Source: CAD feature listing. Evaluate the final solid. Frame: model axes, mm. A direction names the side the tool comes from. Coordinates: 2 decimals unless noted, no trailing zeros. Order: outer loops, then holes, each group sorted by start corner. A loop starts at its lowest first (then second) coordinate and runs counter-clockwise, first axis right, second up.
Item 1: Section B-B on x = 17. Return the cut outline in (y, z), then the cut area to 4 significant figures.
Item 2: Reachability of faces 1 (the flat face through (0, 2, 20)), 2 (the cylindrical face through (-0.74, 10.9, -3.32)), 3 (the flat face through (0, 2, -20)), 4 (the flat face through (0, -3.5, 0)) from +Z, -Z, +X, -X, +Y, -Y: full face, straight path, thin tool, end or side. Return the list, or none.
Item 3: Ray query, line 1 (Y direction, x = -17, z = -22); line 2 (Y direction, x = -10, z = 6.5); line 3 (X direction, y = 10.75, z = -0.5). Return the intervals inside material, ascending.
Item 4: Section A-A on z = 0. Return the cut outline in (x, y), then the cut area to 3 significant figures.
Item 5: Section C-C on y = 1. Return the cut outline in (x, z).
Item 6: Contact query for flat-ended pins moving along their axis: P1, Ø3, axis at x = -9, z = 21, coming from the +Y side; P2, Ø1, axis at x = -2.5, y = 2.5, coming from the -Z side; P3, Ø1, axis at x = -5.5, y = 1.5, coming from the +Z side. Output: stop coordinate, or through.
Item 7: Section D-D on x = 0. Return the cut outline in (y, z).
Autodesk Inventor part; units mm, degrees
ref_plane "YZ Plane" through (0, 0, 0) normal (1, 0, 0) x (0, 1, 0)
ref_plane "XZ Plane" through (0, 0, 0) normal (0, 1, 0) x (-1, 0, 0)
ref_plane "XY Plane" through (0, 0, 0) normal (0, 0, 1) x (1, 0, 0)
sketch "Sketch1" plane through (0, 0, 0) normal (0, 1, 0) x (-1, 0, 0)
  line L0 (20, 20) -> (-20, 20)
  line L1 (-20, 20) -> (-20, -20)
  line L2 (-20, -20) -> (20, -20)
  line L3 (20, -20) -> (20, 20)
  point P0 (0, 0)
  point P1 (20, 0)
  point P2 (0, -20)
  dimension "d0" = 40
  dimension "d1" = 40
extrude "Extrusion1" add sketch "Sketch1" along normal blind 3.5
sketch "Sketch2" plane through (0, 0, 0) normal (0, -1, 0) x (1, 0, 0)
  line L0 (20, 23.5) -> (-20, 23.5)
  line L1 (-20, 23.5) -> (-20, -23.5)
  line L2 (-20, -23.5) -> (20, -23.5)
  line L3 (20, -23.5) -> (20, 23.5)
  line L4 (20, 20) -> (20, -20)
  line L5 (20, -20) -> (-20, -20)
  point P0 (0, 0)
  point P1 (0, -23.5)
  point P2 (20, 0)
  dimension "d5" = 3.5
extrude "Extrusion2" add sketch "Sketch2" along normal blind 3.5
sketch "Sketch3" plane through (0, 3.5, 0) normal (0, 1, 0) x (1, 0, 0)
  line L0 (-12.5, 12.5) -> (12.5, 12.5)
  line L1 (12.5, 12.5) -> (12.5, -12.5)
  line L2 (12.5, -12.5) -> (-12.5, -12.5)
  line L3 (-12.5, -12.5) -> (-12.5, 12.5)
  circle A0 centre (0, 0) radius 3.4
  point P0 (12.5, 0)
  point P1 (0, 12.5)
  dimension "d8" = 25
  dimension "d9" = 25
  dimension "d12" = 6.8
extrude "Extrusion4" add sketch "Sketch3" along normal blind 15 contours A0
properties part number "Einschub"
Answer list:
1. outline: (-3.5, -23.5) - (0, -23.5) - (0, -20) - (3.5, -20) - (3.5, 20) - (0, 20) - (0, 23.5) - (-3.5, 23.5) - close
1. area: 304.5 mm2
2. face 1: +Z, +X, -X, +Y
2. face 2: +Y
2. face 3: -Z, +X, -X, +Y
2. face 4: +Z, -Z, +X, -X, -Y
3. line 1: y = -3.5 to 0
3. line 2: y = -3.5 to 3.5
3. line 3: x = -3.36 to 3.36
4. outline: (-20, -3.5) - (20, -3.5) - (20, 3.5) - (3.4, 3.5) - (3.4, 18.5) - (-3.4, 18.5) - (-3.4, 3.5) - (-20, 3.5) - close
4. area: 382 mm2
5. outline: (-20, -20) - (20, -20) - (20, 20) - (-20, 20) - close
6. P1: stops at y = 3.5
6. P2: stops at z = -20
6. P3: stops at z = 20
7. outline: (-3.5, -23.5) - (0, -23.5) - (0, -20) - (3.5, -20) - (3.5, -3.4) - (18.5, -3.4) - (18.5, 3.4) - (3.5, 3.4) - (3.5, 20) - (0, 20) - (0, 23.5) - (-3.5, 23.5) - close
